from build123d import *

# Parameters (mm, degrees)
ESQUISSE1_R             = 5
BOSS_EXTRU_1_DEPTH      = 4
ESQUISSE2_R             = 3.9
BOSS_EXTRU_2_DEPTH      = 8
CONG_1_R                = 1
ESQUISSE3_R             = 3
ENL_V_MAT_EXTRU_2_DEPTH = 6
ESQUISSE4_W             = 2
ESQUISSE4_H             = 1
BOSS_EXTRU_3_DEPTH      = 5
CONG_2_R                = 0.5


with BuildPart() as part:
    # Esquisse1 → Boss.-Extru.1 (new body)
    with BuildSketch(Plane(origin=(0, 0, 0), x_dir=(1, 0, 0), z_dir=(0, 1, 0))):
        Circle(ESQUISSE1_R)
    extrude(amount=BOSS_EXTRU_1_DEPTH)

    # Esquisse2 → Boss.-Extru.2 (add)
    with BuildSketch(Plane(origin=(0, 4, 0), x_dir=(1, 0, 0), z_dir=(0, 1, 0))):
        Circle(ESQUISSE2_R)
    extrude(amount=BOSS_EXTRU_2_DEPTH)

    # Congé1
    cong_1_edges = [part.edges().sort_by_distance(p)[0] for p in [
        (-5, 0, 0),
    ]]
    fillet(cong_1_edges, radius=CONG_1_R)

    # Esquisse3 → Enlèv. mat.-Extru.2 (cut)
    with BuildSketch(Plane.XZ):
        Circle(ESQUISSE3_R)
    extrude(amount=-ENL_V_MAT_EXTRU_2_DEPTH, mode=Mode.SUBTRACT)

    # Esquisse4 → Boss.-Extru.3 (add)
    with BuildSketch(Plane(origin=(0, 12, 0), x_dir=(1, 0, 0), z_dir=(0, 1, 0))):
        with Locations((0, -2.5)):
            Rectangle(ESQUISSE4_W, ESQUISSE4_H)
        with Locations((0, 2.5)):
            Rectangle(ESQUISSE4_W, ESQUISSE4_H)
    extrude(amount=BOSS_EXTRU_3_DEPTH)

    # Congé2
    cong_2_edges = [part.edges().sort_by_distance(p)[0] for p in [
        (-3.9, 12, 0),
    ]]
    fillet(cong_2_edges, radius=CONG_2_R)


solid = part.part
Work out the finished part from the listing and answer in its coordinate system (mm). A direction names the side the tool comes from. Round coordinates to 2 decimals unless told otherwise and drop trailing zeros. Loops run counter-clockwise (first coordinate to the right, second up) from the corner with the lowest first, then second, coordinate; pieces in that order, holes last. Notation, with made-up numbers: M -23.75,67.5 L 5.25,67.5 A32 ccw 5.25,101.5 Z; hole C 45,78 d4. An arc over 180 degrees is marked long. One line per question, with ' | ' between items. Start each with the question number.
(1) A cutting plane is placed at B-B on x = 0. Write down the section's boundary in (y, z), plus the area to 3 significant figures.
(2) A cutting plane is placed at C-C on y = 3. Write down the section's boundary in (x, z), plus the area to 3 significant figures.
(3) A tool of negligible diameter and unlimited length cuts with its end or side. For faces 1 (the face through (0, 14, 2)), 2 (the face through (-2.87, 7.7, -2.64)), 3 (the face through (0, 6, 0)), 4 (the face through (1, 14.5, 2.5)), 5 (the face through (0, 14, -3)), from which of +Z, -Z, +X, -X, +Y, -Y can it reach the whole face along a straight path? Write none if from no direction.
(4) Find the intervals of material crossed by line 1 (Z direction, x = 0, y = 3.3); line 2 (X direction, y = 1.75, z = -2.5); line 3 (Y direction, x = -0.75, z = -1.5), in increasing order.
(5) A cutting plane is placed at D-D on y = 8. Write down the section's boundary in (x, z).
(6) A cutting plane is placed at A-A on y = 14.25. Write down the section's boundary in (x, z).
(7) Flat-ended cylindrical pins translate along their axes: pin 1 Ø1.1 at (y, z) = (14.5, 2.5) entering from +X; pin 2 Ø3 at (x, z) = (0.5, -0.5) entering from -Y; pin 3 Ø6 at (x, y) = (2, 9) entering from +Z. Find the tip coordinate at first contact, or state that the pin passes through.
(8) For a pull along Z with two mould halves and no side action, classify faces 6 (the face through (-1, 14.5, 2.5)), 7 (the face through (0, 14, 3)), 8 (the face through (0, 14, -2)) as released by +Z, released by -Z, zero draft, split by the parting line, or undercut.
Geometry check:
1) outline: M 0,-4 A1 ccw 1,-5 L 4,-5 L 4,-3.9 L 11.5,-3.9 A0.5 ccw 12,-3.4 L 12,-3 L 17,-3 L 17,-2 L 12,-2 L 12,2 L 17,2 L 17,3 L 12,3 L 12,3.4 A0.5 ccw 11.5,3.9 L 4,3.9 L 4,5 L 1,5 A1 ccw 0,4 L 0,3 L 6,3 L 6,-3 L 0,-3 Z | area: 75.9 mm²
2) outline: C 0,0 d10; hole C 0,0 d6 | area: 50.3 mm²
3) face 1: +X, -X, +Y | face 2: +Y | face 3: -Y | face 4: +Z, -Z, +X, +Y | face 5: -Z, +X, -X, +Y
4) line 1: z = -5 to -3, 3 to 5 | line 2: x = -4.33 to -1.66, 1.66 to 4.33 | line 3: y = 6 to 12
5) outline: C 0,0 d7.8
6) outline: M -1,-3 L 1,-3 L 1,-2 L -1,-2 Z; M -1,2 L 1,2 L 1,3 L -1,3 Z
7) pin 1: stops at x = 1 | pin 2: stops at y = 6 | pin 3: stops at z = 3.9
8) face 6: zero draft | face 7: released by +Z | face 8: undercut
